Geometry: final body of the model. Coordinates: model frame, mm. A direction names the side the tool comes from. Give positions to 0.01 mm unless a question says otherwise; leave off trailing zeros. Order: outer loops, then holes, each group sorted by start corner. A loop starts at its lowest first (then second) coordinate and runs counter-clockwise, first axis right, second up. Notation, with made-up numbers: (34, -4) - (92, -4) arc R23 ccw to (92, 13) - close; hole circle Ø11 at (86, 70.25). An arc over 180 degrees is marked (long way). One line per item, written item: value.
```python
from build123d import *

# Parameters (mm, degrees)
SKETCH1_R           = 17.5
SKETCH1_R_2         = 12.75
BOSS_EXTRUDE1_DEPTH = 175
SKETCH3_R           = 3.25
BOSS_EXTRUDE2_DEPTH = 10


with BuildPart() as part:
    # Sketch1 → Boss-Extrude1 (new, symmetric)
    with BuildSketch(Plane(origin=(0, 0, 0), x_dir=(1, 0, 0), z_dir=(0, 1, 0))):
        with Locations(Location((0, 0, 0), (0, 0, 270))):
            Circle(SKETCH1_R)
        with Locations(Location((0, 0, 0), (0, 0, 270))):
            Circle(SKETCH1_R_2, mode=Mode.SUBTRACT)
    extrude(amount=BOSS_EXTRUDE1_DEPTH, both=True)

    # Sketch3 → Boss-Extrude2 (add)
    # profile 1 of 2: a face of its own
    with BuildSketch(Plane(origin=(0, -55, 0), x_dir=(-1, 0, 0), z_dir=(0, -1, 0))):
        with BuildLine():
            Line((47, -10), (7.90964601, -10))
            ThreePointArc((7.90964601, -10), (12.75, 0), (7.90964601, 10))
            Line((7.90964601, 10), (47, 10))
            Line((47, 10), (47, -10))
        make_face()
        with Locations(Location((30, 0, 0), (0, 0, 270))):
            Circle(SKETCH3_R, mode=Mode.SUBTRACT)
    # profile 2 of 2: a face of its own
    with BuildSketch(Plane(origin=(0, -55, 0), x_dir=(-1, 0, 0), z_dir=(0, -1, 0))):
        with BuildLine():
            Line((-47, -10), (-47, 10))
            Line((-47, 10), (-7.90964601, 10))
            ThreePointArc((-7.90964601, 10), (-12.75, 0), (-7.90964601, -10))
            Line((-7.90964601, -10), (-47, -10))
        make_face()
        with Locations(Location((-30, 0, 0), (0, 0, 90))):
            Circle(SKETCH3_R, mode=Mode.SUBTRACT)
    extrude(amount=-BOSS_EXTRUDE2_DEPTH)


solid = part.part
```
1) Section C-C, the plane y = -74. Return loops of the section in (x, z), then the cut area to 3 significant figures.
Answers below:
outline: circle Ø35 at (0, 0); hole circle Ø25.5 at (0, 0)
area: 451 mm^2
2) Mould query, pull axis X, two halves, no side actions, for faces 6 (the face through (30, -50, 10)), 7 (the face through (-47, -50, 0)), 8 (the face through (26.827, -50.07, 0.705)). Classes: released by +X, released by -X, zero draft, split by the parting line, or undercut.
Answers below:
face 6: zero draft
face 7: released by -X
face 8: undercut
3) Section B-B, the plane z = 0. Return loops of the section in (x, y), then the cut area to 4 significant figures.
Answers below:
outline: (-47, -55) - (-33.25, -55) - (-33.25, -45) - (-47, -45) - close; (-26.75, -55) - (-17.5, -55) - (-17.5, -175) - (-12.75, -175) - (-12.75, 175) - (-17.5, 175) - (-17.5, -45) - (-26.75, -45) - close; (12.75, -175) - (17.5, -175) - (17.5, -55) - (26.75, -55) - (26.75, -45) - (17.5, -45) - (17.5, 175) - (12.75, 175) - close; (33.25, -55) - (47, -55) - (47, -45) - (33.25, -45) - close
area: 3,785 mm^2
4) Set-up query: faces 1 (the face through (-13, 175, 1)), 2 (the face through (-31, -50, 10)), 3 (the face through (31, -50, -10)), 4 (the face through (-30, -50, -10)), 5 (the face through (-10.648, 2.45, -13.887)). Return all of +Z, -Z, +X, -X, +Y, -Y with unobstructed straight access to the full face (end or side cutting, diameter ignored); none if empty.
Answers below:
face 1: +Z, -Z, +X, -X, +Y
face 2: +Z, -X, +Y, -Y
face 3: -Z, +X, +Y, -Y
face 4: -Z, -X, +Y, -Y
face 5: none
5) Material intervals for line 1 along X through (y, z) = (-50.75, 0); line 2 along X through (y, z) = (82, 0); line 3 along Z through (x, y) = (-30, -48.5), sorted ascending.
Answers below:
line 1: -47 to -33.25, -26.75 to -12.75, 12.75 to 26.75, 33.25 to 47
line 2: -17.5 to -12.75, 12.75 to 17.5
line 3: -10 to -3.25, 3.25 to 10
6) First-contact query: pin 1 (11 mm diameter, centred on x = -37, y = -48.5, fed in from +Z); pin 2 (1 mm diameter, centred on x = -16, y = 74, fed in from -Z); pin 3 (1.5 mm diameter, centred on x = 12.5, y = 27, fed in from -Z); pin 4 (6 mm diameter, centred on x = -30, z = 0, fed in from -Y). Flat tips, straight axial feed; report the tip coordinate or a pass-through.
Answers below:
pin 1: z = 10
pin 2: z = -8.12
pin 3: z = -12.97
pin 4: through
7) Section D-D, the plane x = 30. Return loops of the section in (y, z).
Answers below:
outline: (-55, -10) - (-45, -10) - (-45, -3.25) - (-55, -3.25) - close; (-55, 3.25) - (-45, 3.25) - (-45, 10) - (-55, 10) - close
8) Section A-A, the plane x = 0. Return loops of the section in (y, z), then the cut area to 4 significant figures.
Answers below:
outline: (-175, -17.5) - (175, -17.5) - (175, -12.75) - (-175, -12.75) - close; (-175, 12.75) - (175, 12.75) - (175, 17.5) - (-175, 17.5) - close
area: 3,325 mm^2
